from build123d import *

# Parameters (mm, degrees)
SKETCH1_R               = 12.5
SKETCH1_R_2             = 5.5
BOSS_EXTRUDE1_DEPTH     = 50
SKETCH3_R               = 5.5
CUT_EXTRUDE2_DEPTH      = 6
BOSS_EXTRUDE2_DEPTH     = 10
CUT_EXTRUDE3_REACH      = 177.357
CUT_EXTRUDE3_END_RADIUS = 31
SKETCH8_R               = 12.5
SKETCH8_R_2             = 3.3
SKETCH9_R               = 5.5
CUT_EXTRUDE4_DEPTH      = 6
SKETCH11_R              = 3.3
CUT_EXTRUDE5_DEPTH      = 170.437304068


with BuildPart() as part:
    # Sketch1 → Boss-Extrude1 (new body)
    # profile 1 of 3: a face of its own
    with BuildSketch(Plane.XY):
        with BuildLine():
            ThreePointArc((93.048941287, 25.965408086), (94.65877554, 21.378133023), (97.956410185, 17.805981771))
            ThreePointArc((97.956410185, 17.805981771), (90.215500805, 14.226887077), (81.775930618, 13))
            Line((81.775930618, 13), (0, 13))
            Line((0, 13), (0, 0))
            Line((0, 0), (50, 0))
            Line((50, 0), (50, 3))
            Line((50, 3), (81.775930618, 3))
            ThreePointArc((81.775930618, 3), (100.673195021, 7.794200226), (114.99953828, 21.017166857))
            Line((114.99953828, 21.017166857), (126.762369546, 39.090235236))
            ThreePointArc((126.762369546, 39.090235236), (129.32062945, 44.831511086), (129.970641881, 51.083264917))
            Line((129.970641881, 51.083264917), (128.838231587, 71.959931438))
            ThreePointArc((128.838231587, 71.959931438), (120.710453355, 83.318007797), (107.33724849, 79.290096524))
            Line((107.33724849, 79.290096524), (94.165028172, 62.21694181))
            ThreePointArc((94.165028172, 62.21694181), (90.681483474, 55.176380902), (90.178041223, 47.33730395))
            Line((90.178041223, 47.33730395), (93.048941287, 25.965408086))
        make_face()
        with Locations((110, 50)):
            Circle(SKETCH1_R, mode=Mode.SUBTRACT)
        with Locations((116.838231587, 71.959931438)):
            Circle(SKETCH1_R_2, mode=Mode.SUBTRACT)
        with Locations((104.942116553, 27.563025716)):
            Circle(SKETCH1_R_2, mode=Mode.SUBTRACT)
    # profile 2 of 3: a face of its own
    with BuildSketch(Plane.XY):
        with Locations((116.838231587, 71.959931438)):
            Circle(SKETCH1_R_2)
    # profile 3 of 3: a face of its own
    with BuildSketch(Plane.XY):
        with Locations((104.942116553, 27.563025716)):
            Circle(SKETCH1_R_2)
    extrude(amount=BOSS_EXTRUDE1_DEPTH)

    # Sketch3 → Cut-Extrude2 (cut)
    with BuildSketch(Plane.XY.offset(50)):
        with Locations((116.838231587, 71.959931438)):
            Circle(SKETCH3_R)
        with Locations((104.942116553, 27.563025716)):
            Circle(SKETCH3_R)
    extrude(amount=-CUT_EXTRUDE2_DEPTH, mode=Mode.SUBTRACT)

    # Sketch5 → Boss-Extrude2 (add)
    with BuildSketch(Plane(origin=(0, 0, 0), x_dir=(-1, 0, 0), z_dir=(0, 0, -1))):
        with BuildLine():
            Line((-81.775930618, 13), (0, 13))
            Line((0, 13), (0, 20))
            ThreePointArc((0, 20), (-5.857864376, 34.142135624), (-20, 40))
            Line((-20, 40), (-76.458980338, 40))
            Line((-76.458980338, 40), (-80.657198498, 40))
            Line((-80.657198498, 40), (-91.163665826, 40))
            Line((-91.163665826, 40), (-93.048941287, 25.965408086))
            ThreePointArc((-93.048941287, 25.965408086), (-94.65877554, 21.378133023), (-97.956410185, 17.805981771))
            ThreePointArc((-97.956410185, 17.805981771), (-90.215500805, 14.226887077), (-81.775930618, 13))
        make_face()
    extrude(amount=-BOSS_EXTRUDE2_DEPTH)

    # Sketch6 → Revolve2 (revolve)
    with BuildSketch(Plane.ZY.offset(-110), mode=Mode.PRIVATE) as revolve2_sk:
        with BuildLine():
            ThreePointArc((31, 50), (21.920310217, 71.920310217), (0, 81))
            Line((0, 81), (0, 50))
            Line((0, 50), (31, 50))
        make_face()
        with BuildLine():
            Line((0, 85), (0, 81))
            ThreePointArc((0, 81), (21.920310217, 71.920310217), (31, 50))
            Line((31, 50), (35, 50))
            ThreePointArc((35, 50), (24.748737342, 74.748737342), (0, 85))
        make_face()
    revolve(revolve2_sk.sketch.rotate(Axis((110, 50, 35), (0, 0, -1)), 270), axis=Axis((110, 50, 35), (0, 0, -1)))

    # Sketch6<5> → Cut-Revolve3 (revolve, cut)
    with BuildSketch(Plane.ZY.offset(-110)):
        with BuildLine():
            ThreePointArc((31, 50), (21.920310217, 71.920310217), (0, 81))
            Line((0, 81), (0, 50))
            Line((0, 50), (31, 50))
        make_face()
    revolve(axis=Axis((110, 50, 35), (0, 0, -1)), mode=Mode.SUBTRACT)

    # Cut-Extrude3: up to this sphere (the profile starts outside it)
    cut_extrude3_end = Location((110, 50, 0)) * Sphere(CUT_EXTRUDE3_END_RADIUS, mode=Mode.PRIVATE)
    # Sketch8 → Cut-Extrude3 (cut, up to the surface)
    with BuildSketch(Plane.XY.offset(50), mode=Mode.PRIVATE) as cut_extrude3_sk1:
        with Locations(Location((110, 50, 0), (0, 0, 180))):
            Circle(SKETCH8_R)
    cut_extrude3_tool1 = extrude(cut_extrude3_sk1.sketch, amount=-CUT_EXTRUDE3_REACH, mode=Mode.PRIVATE) - cut_extrude3_end
    add(cut_extrude3_tool1.solids().sort_by_distance((110, 50, 50))[0], mode=Mode.SUBTRACT)
    # Sketch8 → Cut-Extrude3 (cut, up to the surface)
    with BuildSketch(Plane.XY.offset(50), mode=Mode.PRIVATE) as cut_extrude3_sk2:
        with Locations((116.838231587, 71.959931438)):
            Circle(SKETCH8_R_2)
    cut_extrude3_tool2 = extrude(cut_extrude3_sk2.sketch, amount=-CUT_EXTRUDE3_REACH, mode=Mode.PRIVATE) - cut_extrude3_end
    add(cut_extrude3_tool2.solids().sort_by_distance((116.838232, 71.959931, 50))[0], mode=Mode.SUBTRACT)
    # Sketch8 → Cut-Extrude3 (cut, up to the surface)
    with BuildSketch(Plane.XY.offset(50), mode=Mode.PRIVATE) as cut_extrude3_sk3:
        with Locations((104.942116553, 27.563025716)):
            Circle(SKETCH8_R_2)
    cut_extrude3_tool3 = extrude(cut_extrude3_sk3.sketch, amount=-CUT_EXTRUDE3_REACH, mode=Mode.PRIVATE) - cut_extrude3_end
    add(cut_extrude3_tool3.solids().sort_by_distance((104.942117, 27.563026, 50))[0], mode=Mode.SUBTRACT)

    # Sketch9 → Cut-Extrude4 (cut)
    with BuildSketch(Plane(origin=(0, 13, 0), x_dir=(1, 0, 0), z_dir=(0, 1, 0))):
        with Locations(Location((15.190815531, -40, 0), (0, 0, 180))):
            Circle(SKETCH9_R)
        with Locations(Location((35.190815531, -20, 0), (0, 0, 180))):
            Circle(SKETCH9_R)
    extrude(amount=-CUT_EXTRUDE4_DEPTH, mode=Mode.SUBTRACT)

    # Sketch11 → Cut-Extrude5 (cut, through all)
    with BuildSketch(Plane(origin=(0, 13, 0), x_dir=(1, 0, 0), z_dir=(0, 1, 0))):
        with Locations(Location((35.190815531, -20, 0), (0, 0, 180))):
            Circle(SKETCH11_R)
        with Locations(Location((15.190815531, -40, 0), (0, 0, 180))):
            Circle(SKETCH11_R)
    extrude(amount=-CUT_EXTRUDE5_DEPTH, mode=Mode.SUBTRACT)


solid = part.part
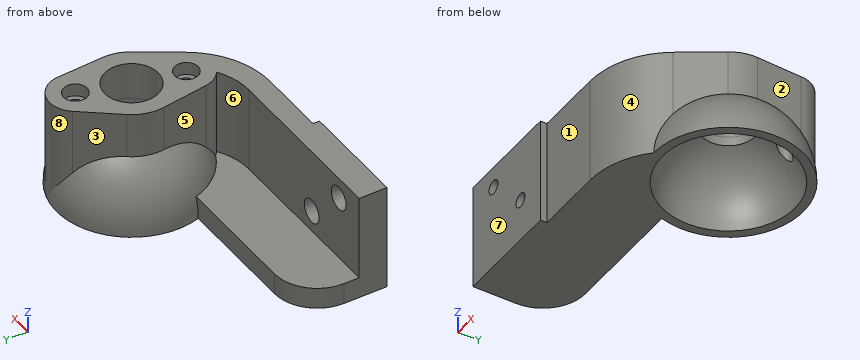
Check sheet for the modelled part. Datum: model origin and axes. Units: mm. Face numbers are marked on the shaded views. A direction names the side the tool comes from. Coordinates: 2 decimals unless noted, no trailing zeros. Write each loop counter-clockwise with the first axis right and the second up, starting at its lowest first coordinate (ties: lowest second). Pieces come first, ordered by that corner, then holes.
Item 1: Cross-section at B-B on z = 40. Record the boundary of the cut face in (x, y).
Numbers:
outline: (0, 0) - (11.89, 0) - (11.89, 7) - (9.69, 7) - (9.69, 13) - (0, 13) - close; (18.49, 0) - (50, 0) - (50, 3) - (81.78, 3) arc R39.64 ccw to (115, 21.02) - (126.76, 39.09) arc R20 ccw to (129.97, 51.08) - (128.84, 71.96) arc R12 ccw to (107.34, 79.29) - (94.17, 62.22) arc R20 ccw to (90.18, 47.34) - (93.05, 25.97) arc R12 ccw to (97.96, 17.81) arc R29.64 cw to (81.78, 13) - (20.69, 13) - (20.69, 7) - (18.49, 7) - close; hole circle Ø25 at (110, 50); hole circle Ø6.6 at (104.94, 27.56); hole circle Ø6.6 at (116.84, 71.96)
Item 2: Depth check by flat-ended pin: pin 1 Ø2 at (x, z) = (129, 41) entering from -Y; pin 2 Ø3.5 at (x, y) = (119, 72.5) entering from +Z; pin 3 Ø6 at (y, z) = (75, 34.5) entering from -X; pin 4 Ø4 at (x, z) = (15.19, 40) entering from +Y. Enter the tip coordinate at first touch or a pass-through.
Numbers:
pin 1: stops at y = 41.28
pin 2: stops at z = 44
pin 3: stops at x = 101.71
pin 4: passes through
Item 3: Access from +Z, -Z, +X, -X, +Y, -Y to the whole of each face (thin tool, end or side, straight path). Record for the marked faces 1, 2, 3, 4 and 5.
Numbers:
face 1: +Z, -Z, +X, -Y
face 2: +Z, +X, +Y
face 3: +Z, -X, +Y
face 4: +Z, +X, -Y
face 5: +Z, -X
Item 4: Cross-section at C-C on x = 14.5. Record the boundary of the cut face in (y, z), then the cut area to 3 significant figures.
Numbers:
outline: (0, 0) - (39.23, 0) - (39.23, 10) - (13, 10) - (13, 34.54) - (7, 34.54) - (7, 36.77) - (0, 36.77) - close; (0, 43.23) - (7, 43.23) - (7, 45.46) - (13, 45.46) - (13, 50) - (0, 50) - close
area: 802 mm2
Item 5: Mould release check, pull along Y, two halves, no side actions. Record for the marked faces 6, 7 and 8: released by +Y, released by -Y, zero draft, split by the parting line, or undercut.
Numbers:
face 6: undercut
face 7: released by -Y
face 8: released by +Y
Item 6: Cross-section at A-A on x = 117. Record the boundary of the cut face in (y, z), then the cut area to 3 significant figures.
Numbers:
outline: (15.71, 0) - (19.8, 0) arc R30.2 cw to (39.64, 28.37) - (39.64, 50) - (24.09, 50) - (24.09, 22.47) arc R34.29 ccw to start; (60.36, 28.37) arc R30.2 cw to (68.66, 23.74) - (68.66, 44) - (66.46, 44) - (66.46, 50) - (60.36, 50) - close; (75.26, 16.56) arc R30.2 cw to (80.2, 0) - (84.29, 0) arc R34.29 ccw to (83.96, 4.77) - (83.96, 50) - (77.46, 50) - (77.46, 44) - (75.26, 44) - close
area: 1,050 mm2
Item 7: Scan lines: probe 1 along Z at (x, y) = (30.5, 24); probe 2 along Y at (x, z) = (93, 19); probe 3 along X at (y, z) = (58, 13). Record each from-to range of solid material in increasing order.
Numbers:
probe 1: z = 0 to 10
probe 2: y = 4.62 to 15.21, 26.02 to 32.36, 67.64 to 73.98
probe 3: x = 78.5 to 83.02, 136.98 to 141.5
Item 8: Cross-section at D-D on y = 36. Record the boundary of the cut face in (x, z).
Numbers:
outline: (8, 0) - (82.34, 0) arc R27.66 cw to (137.66, 0) - (142.08, 0) arc R32.08 ccw to (124.75, 28.49) - (124.75, 50) - (91.7, 50) - (91.7, 26.35) arc R32.08 ccw to (79.52, 10) - (8, 10) - close
